from build123d import *

# Parameters (mm, degrees)
F0_R     = 10
F1_DEPTH = 2000
F2_R     = 2
F3_DEPTH = 12.5


with BuildPart() as f1:
    # F0 (on Top) → F1 (new body)
    with BuildSketch(Plane.XY):
        Circle(F0_R)
    extrude(amount=F1_DEPTH)

    # F2 (on Right) → F3 (cut, symmetric)
    with BuildSketch(Plane.YZ):
        with Locations((0, 198)):
            Circle(F2_R)
        with Locations((0, 358)):
            Circle(F2_R)
        with Locations((0, 518)):
            Circle(F2_R)
        with Locations((0, 678)):
            Circle(F2_R)
        with Locations((0, 838)):
            Circle(F2_R)
        with Locations((0, 998)):
            Circle(F2_R)
        with Locations((0, 1158)):
            Circle(F2_R)
        with Locations((0, 1318)):
            Circle(F2_R)
        with Locations((0, 1478)):
            Circle(F2_R)
        with Locations((0, 1638)):
            Circle(F2_R)
    extrude(amount=F3_DEPTH, both=True, mode=Mode.SUBTRACT)


solid = f1.part
The model under review builds one solid part; all positions refer to its coordinate system, in mm. Round coordinates to 2 decimals unless told otherwise and drop trailing zeros. Write each loop counter-clockwise with the first axis right and the second up, starting at its lowest first coordinate (ties: lowest second). Pieces come first, ordered by that corner, then holes. Notation, with made-up numbers: (-33.5, 46.25) - (-2.5, 46.25) arc R16 ccw to (-2.5, 69.25) - close; hole circle Ø5 at (88.25, 84). An arc over 180 degrees is marked (long way). One line per item, written item: value. Start each with the question number.
1. To check wall thickness, follow L1, parallel to Y at x = -2.25, z = 838; L2, parallel to X at y = -2, z = 1857; L3, parallel to Y at x = 0.5, z = 1408. State the ranges of each line that lie inside material, in increasing order. Write a range as from..to.
2. Clearance check with flat-ended pins moving along their axes: P1, Ø6.5, axis at y = 0, z = 1638, coming from the -X side; P2, Ø8, axis at x = 6.5, z = 1629.5, coming from the +Y side; P3, Ø8, axis at y = -5.5, z = 596.5, coming from the -X side; P4, Ø5, axis at y = 7, z = 1037.5, coming from the +X side. State where each tip first meets the part, or that it passes through.
3. Consider section A-A on z = 1797.5. Write out the cut boundary in (x, y), and give its area (3 significant figures).
Checks:
1. L1: y = -9.74..-2, 2..9.74
1. L2: x = -9.8..9.8
1. L3: y = -9.99..9.99
2. P1: stops at x = -10
2. P2: stops at y = 9.68
2. P3: stops at x = -9.89
2. P4: stops at x = 8.93
3. outline: circle Ø20 at (0, 0)
3. area: 314 mm^2
